Geometry: see drawing. Coordinates: mm, zero at the bounding-box minimum. A direction names the side the tool comes from. Coordinates: 2 decimals unless noted, no trailing zeros. Write each loop counter-clockwise with the first axis right and the second up, starting at its lowest first coordinate (ties: lowest second). Pieces come first, ordered by that corner, then holes. Notation, with made-up numbers: M -5,25 L 4,25 A21 ccw 4,51 Z; hole C 36,-29 d4. An arc over 180 degrees is marked long. One line per item, written item: value. Start each with the question number.
Item 1: Cut plane A-A, the plane x = 38.1. State how many separate pieces and enclosed holes the cut face has.
Item 2: Cut plane B-B, the plane z = 60.5. Output: boundary loops of the cut face in (x, y) (1 decimal).
Item 3: Pin query (flat end, axial travel): P1, Ø4, axis at x = 59.75, z = 46.49, coming from the +Y side; P2, Ø23, axis at x = 52, z = 75, coming from the +Y side; P3, Ø8.5, axis at x = 38.1, z = 83.99, coming from the -Y side. Return the tip coordinate at first contact, or that it passes through.
Item 4: Cut plane D-D, the plane z = 30. Output: boundary loops of the cut face in (x, y) (1 decimal).
Item 5: Set-up query: the marked faces 1 and 2. Return all of +Z, -Z, +X, -X, +Y, -Y with unobstructed straight access to the full face (end or side cutting, diameter ignored); none if empty.
Item 6: Ray query, L1, parallel to Z at x = 38.1, y = 5; L2, parallel to Z at x = 16.5, y = 4; L3, parallel to Y at x = 42, z = 7 (1 decimal). Return the intervals inside material, ascending. Write a range as from..to.
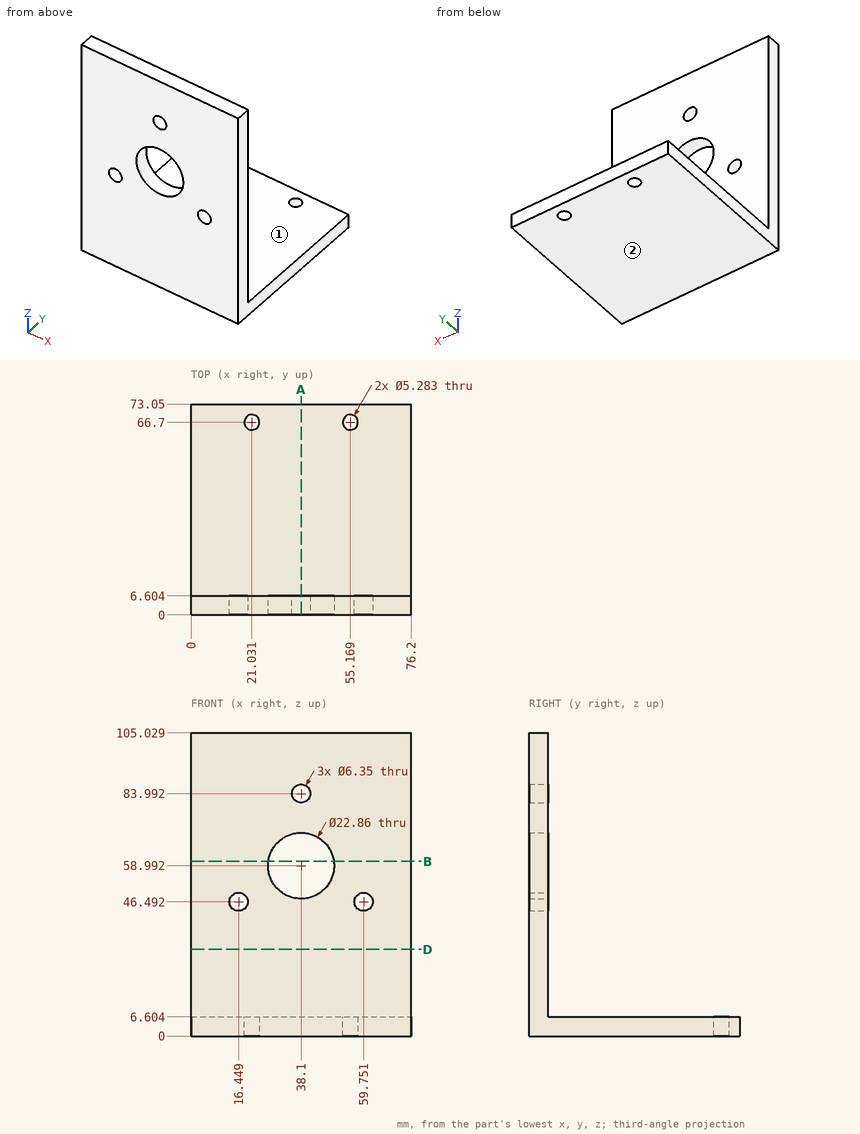
From the geometry:
1. separate pieces: 3
1. enclosed holes: 0
2. outline: M 0,0 L 26.8,0 L 26.8,6.6 L 0,6.6 Z; M 49.4,0 L 76.2,0 L 76.2,6.6 L 49.4,6.6 Z
3. P1: passes through
3. P2: stops at y = 6.6
3. P3: stops at y = 0
4. outline: M 0,0 L 76.2,0 L 76.2,6.6 L 0,6.6 Z
5. face 1: +Z, +X, -X, +Y
5. face 2: -Z, +X, -X, +Y, -Y
6. L1: z = 0..47.56, 70.42..80.82, 87.17..105.03
6. L2: z = 0..43.32, 49.67..105.03
6. L3: y = 0..6.6
